Geometry: final body of the model. Coordinates: model frame, mm. Face numbers are marked on the shaded views. A direction names the side the tool comes from. Round coordinates to 2 decimals unless told otherwise and drop trailing zeros. Loops run counter-clockwise (first coordinate to the right, second up) from the corner with the lowest first, then second, coordinate; pieces in that order, holes last. Notation, with made-up numbers: (8.25, 4.5) - (33.25, 4.5) arc R23 cw to (33.25, 42.5) - close; hole circle Ø3 at (-13.75, -27). An arc over 180 degrees is marked (long way). Answer as a JSON object with one key per item and string values. Group by question number.
Item 1: Section A-A (z = 9). Return the cut outline in (x, y).
Item 2: Line query: line 1 (Y direction, x = -1.5, z = 6.25); line 2 (X direction, y = 0.5, z = 3.5); line 3 (Y direction, x = 3, z = 1.75). Output: solid intervals per line, ascending.
Item 3: Section D-D (z = 1). Return the cut outline in (x, y).
Item 4: Section B-B (x = -1.5). Return the cut outline in (y, z), plus the area to 3 significant figures.
Item 5: Section C-C (y = 0.75). Return the cut outline in (x, z).
Item 6: Draft query along Y for the marked faces 4, 5 and 6. Return one class per face: released by +Y, released by -Y, zero draft, split by the parting line, or undercut.
Item 7: First-contact query: pin 1 (5 mm diameter, centred on x = -8.5, z = 8.5, fed in from -Y); pin 2 (5 mm diameter, centred on x = 5.5, z = 5.5, fed in from +Y); pin 3 (1 mm diameter, centred on y = 3.5, z = 7.5, fed in from -X). Flat tips, straight axial feed; report the tip coordinate or a pass-through.
Item 8: Reachability of the marked faces 1, 2 and 3 from +Z, -Z, +X, -X, +Y, -Y: full face, straight path, thin tool, end or side. Return the list, or none.
```python
from build123d import *

# Parameters (mm, degrees)
SKETCH_1_W      = 35
SKETCH_1_H      = 15
SKETCH_1_W_2    = 18
SKETCH_1_H_2    = 10
EXTRUDE_1_DEPTH = 2
SKETCH_2_W      = 21
SKETCH_2_H      = 13
SKETCH_2_W_2    = 18
SKETCH_2_H_2    = 10
EXTRUDE_2_DEPTH = 10
FILLET_1_R      = 3
FILLET_2_R      = 2
FILLET_3_R      = 2


with BuildPart() as part:
    # 草图1 → 凸台-拉伸1 (new body)
    with BuildSketch(Plane.XY):
        Rectangle(SKETCH_1_W, SKETCH_1_H)
        Rectangle(SKETCH_1_W_2, SKETCH_1_H_2, mode=Mode.SUBTRACT)
    extrude(amount=EXTRUDE_1_DEPTH)

    # 草图2 → 凸台-拉伸2 (add)
    with BuildSketch(Plane.XY.offset(2)):
        Rectangle(SKETCH_2_W, SKETCH_2_H)
        Rectangle(SKETCH_2_W_2, SKETCH_2_H_2, mode=Mode.SUBTRACT)
    extrude(amount=EXTRUDE_2_DEPTH)

    # 圆角1
    fillet_1_edges = [part.edges().sort_by_distance(p)[0] for p in [
        (17.5, -7.5, 1),
        (-17.5, -7.5, 1),
        (-17.5, 7.5, 1),
        (17.5, 7.5, 1),
    ]]
    fillet(fillet_1_edges, radius=FILLET_1_R)

    # 圆角2
    fillet_2_edges = [part.edges().sort_by_distance(p)[0] for p in [
        (9, -5, 6),
        (9, 5, 6),
        (-9, 5, 6),
        (-9, -5, 6),
    ]]
    fillet(fillet_2_edges, radius=FILLET_2_R)

    # 圆角3
    fillet_3_edges = [part.edges().sort_by_distance(p)[0] for p in [
        (10.5, -6.5, 7),
        (10.5, 6.5, 7),
        (-10.5, 6.5, 7),
        (-10.5, -6.5, 7),
    ]]
    fillet(fillet_3_edges, radius=FILLET_3_R)


solid = part.part
```
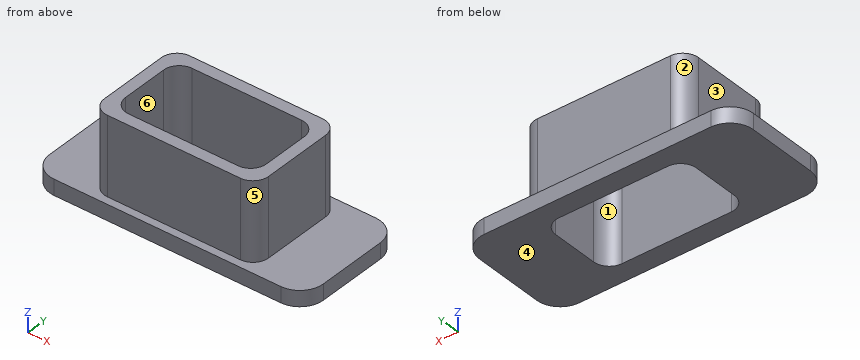
Values:
{
 "1": {"outline": "(-10.5, -4.5) arc R2 ccw to (-8.5, -6.5) - (8.5, -6.5) arc R2 ccw to (10.5, -4.5) - (10.5, 4.5) arc R2 ccw to (8.5, 6.5) - (-8.5, 6.5) arc R2 ccw to (-10.5, 4.5) - close; hole (-9, -3) arc R2 ccw to (-7, -5) - (7, -5) arc R2 ccw to (9, -3) - (9, 3) arc R2 ccw to (7, 5) - (-7, 5) arc R2 ccw to (-9, 3) - close"},
 "2": {"line 1": "y = -6.5 to -5, 5 to 6.5", "line 2": "x = -10.5 to -9, 9 to 10.5", "line 3": "y = -7.5 to -5, 5 to 7.5"},
 "3": {"outline": "(-17.5, -4.5) arc R3 ccw to (-14.5, -7.5) - (14.5, -7.5) arc R3 ccw to (17.5, -4.5) - (17.5, 4.5) arc R3 ccw to (14.5, 7.5) - (-14.5, 7.5) arc R3 ccw to (-17.5, 4.5) - close; hole (-9, -3) arc R2 ccw to (-7, -5) - (7, -5) arc R2 ccw to (9, -3) - (9, 3) arc R2 ccw to (7, 5) - (-7, 5) arc R2 ccw to (-9, 3) - close"},
 "4": {"outline": "(-7.5, 0) - (-5, 0) - (-5, 12) - (-6.5, 12) - (-6.5, 2) - (-7.5, 2) - close; (5, 0) - (7.5, 0) - (7.5, 2) - (6.5, 2) - (6.5, 12) - (5, 12) - close", "area": "40.0 mm^2"},
 "5": {"outline": "(-17.5, 0) - (-9, 0) - (-9, 12) - (-10.5, 12) - (-10.5, 2) - (-17.5, 2) - close; (9, 0) - (17.5, 0) - (17.5, 2) - (10.5, 2) - (10.5, 12) - (9, 12) - close"},
 "6": {"face 4": "zero draft", "face 5": "released by -Y", "face 6": "undercut"},
 "7": {"pin 1": "stops at y = -6.5", "pin 2": "stops at y = 6.5", "pin 3": "stops at x = -10.5"},
 "8": {"face 1": "+Z, -Z", "face 2": "+Z, -X, +Y", "face 3": "+Z, -X, +Y, -Y"}
}
